The model under review builds one solid part; all positions refer to its coordinate system, in mm. Face numbers are marked on the shaded views. A direction names the side the tool comes from. Give positions to 0.01 mm unless a question says otherwise; leave off trailing zeros. Order: outer loops, then holes, each group sorted by start corner. A loop starts at its lowest first (then second) coordinate and runs counter-clockwise, first axis right, second up. Notation, with made-up numbers: (30.25, 89.25) - (66.25, 89.25) arc R14 ccw to (66.25, 115.25) - close; hole circle Ø6 at (15.5, -5.5). An arc over 180 degrees is marked (long way). Use CSV: the item, a comma, the result in double quotes.
```python
from build123d import *

# Parameters (mm, degrees)
CUT_EXTRUDE_1_DEPTH      = 101.359354322
CUT_EXTRUDE_1_DEPTH_BACK = 101.359354322
SKETCH_2_R               = 2


with BuildPart() as part:
    # 草图1 → 旋转1 (revolve)
    with BuildSketch(Plane.XY, mode=Mode.PRIVATE) as revolve_1_sk:
        Polygon((0, 0), (0, 5), (15, 5), (15, 4), (18, 4), (18, 6), (90, 6), (90, 4), (92, 4), (92, 5), (100, 5), (100, 0), align=None)
    revolve(revolve_1_sk.sketch.rotate(Axis((0, 0, 0), (1, 0, 0)), 90), axis=Axis((0, 0, 0), (1, 0, 0)))

    # 草图2 → 切除-拉伸1 (cut, two sides: drawn at the far end of the back side and taken through both)
    with BuildSketch(Plane.XY.offset(-CUT_EXTRUDE_1_DEPTH_BACK)):
        with Locations((10, 0)):
            Circle(SKETCH_2_R)
    extrude(amount=CUT_EXTRUDE_1_DEPTH + CUT_EXTRUDE_1_DEPTH_BACK, mode=Mode.SUBTRACT)

    # 草图4 → 切除-旋转1 (revolve, cut)
    with BuildSketch(Plane(origin=(95, 0, 0), x_dir=(0, 0, -1), z_dir=(1, 0, 0))):
        Polygon((-2.121320344, -2.121320344), (-2.121320344, -4.949747468), (-3.535533906, -3.535533906), align=None)
    revolve(axis=Axis((95, 0, 0), (0, -0.7071067811865489, 0.7071067811865462)), mode=Mode.SUBTRACT)


solid = part.part
```
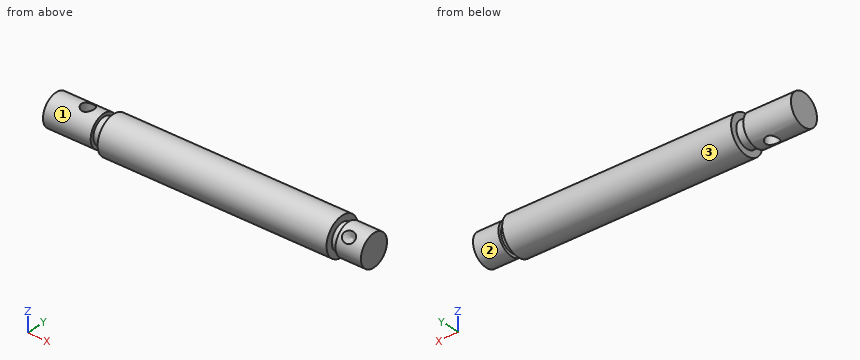
Item 1: Take a section at A-A, the plane z = 0. Give the boundary of the cut face in (x, y).
Results list:
outline,"(0, -5) - (15, -5) - (15, -4) - (18, -4) - (18, -6) - (90, -6) - (90, -4) - (92, -4) - (92, -5) - (100, -5) - (100, 5) - (92, 5) - (92, 4) - (90, 4) - (90, 6) - (18, 6) - (18, 4) - (15, 4) - (15, 5) - (0, 5) - close; hole circle Ø4 at (10, 0)"
Item 2: Take a section at C-C, the plane x = 10. Give the boundary of the cut face in (y, z).
Results list:
outline,"(-2, -4.58) - (-2, 4.58) arc R5 ccw to start; (2, -4.58) arc R5 ccw to (2, 4.58) - close"
Item 3: Take a section at D-D, the plane x = 42. Give the boundary of the cut face in (y, z).
Results list:
outline,"circle Ø12 at (0, 0)"
Item 4: Take a section at B-B, the plane y = 0. Give the boundary of the cut face in (x, z).
Results list:
outline,"(0, -5) - (8, -5) - (8, 5) - (0, 5) - close; (12, -5) - (15, -5) - (15, -4) - (18, -4) - (18, -6) - (90, -6) - (90, -4) - (92, -4) - (92, -5) - (100, -5) - (100, 5) - (92, 5) - (92, 4) - (90, 4) - (90, 6) - (18, 6) - (18, 4) - (15, 4) - (15, 5) - (12, 5) - close"
Item 5: Tool access review of the marked faces 1, 2 and 3: name each direction out of +Z, -Z, +X, -X, +Y, -Y from which nothing blocks a thin tool from reaching the whole face with its end or side.
Results list:
face 1,"-X"
face 2,"+X"
face 3,"+X, -X"
Item 6: Clearance check with flat-ended pins moving along their axes: pin 1 (3 mm diameter, centred on x = 42.5, z = -3, fed in from +Y); pin 2 (6.5 mm diameter, centred on x = 10, y = 0, fed in from -Z); pin 3 (4 mm diameter, centred on x = 31.5, y = -2.5, fed in from +Z). State where each tip first meets the part, or that it passes through.
Results list:
pin 1,"stops at y = 5.81"
pin 2,"stops at z = -5"
pin 3,"stops at z = 5.98"
Item 7: Wall thickness on L1, parallel to X at y = -4.5, z = -0.75; L2, parallel to X at y = 0, z = 2.5; L3, parallel to Y at x = 10, z = 3: over which ranges is each line inside the solid? List them lowest first.
Results list:
L1,"x = 0 to 15, 18 to 90, 92 to 100"
L2,"x = 0 to 8, 12 to 100"
L3,"y = -4 to -2, 2 to 4"
